Read the model definition and answer for the solid it produces. Units are mm, in the model's axes. A direction names the side the tool comes from. Give positions to 0.01 mm unless a question says otherwise; leave off trailing zeros. Loops run counter-clockwise (first coordinate to the right, second up) from the corner with the lowest first, then second, coordinate; pieces in that order, holes last. Notation, with made-up numbers: (70, 65) - (126, 65) arc R31 cw to (126, 93) - close; hole circle Ø9 at (87.25, 89). An arc over 180 degrees is marked (long way). Write each question's results on one line, items separated by ' | '. Start each with the question number.
Q1. The part is cut by section A-A, the plane y = 5. Write down the section's boundary in (x, z) (3 decimals), plus the area to 3 significant figures.
Q2. Given pin 1 (1 mm diameter, centred on x = -8.5, y = -4.5, fed in from +Z), flat-ended and moving along its own axis, determine where the tip first touches the part or whether it passes through.
Q3. Find the intervals of material crossed by line 1 (Y direction, x = -5.5, z = 471.5) (3 decimals), in increasing order. Write a range as from..to.
Q4. Determine the mould class of faces 3 (the flat face through (0, -9.525, 375)), 4 (the flat face through (11, 0, 774.7)), 5 (the flat face through (-12.7, 0, 375)), 6 (the flat face through (-9.525, 0, 375)) for opening direction X: +X half, -X half, draft (parallel to the pull), parting line (faces both ways), or undercut.
Q5. The part is cut by section C-C, the plane z = 679. Write down the section's boundary in (x, y) (3 decimals), plus the area to 3 significant figures.
Q6. For faces 1 (the flat face through (0, 12.7, 375)), 2 (the flat face through (0, 9.525, 375)), determine the directions among +Z, -Z, +X, -X, +Y, -Y from which every point of the face is accessible in a straight line to the end or side of a thin tool.
Autodesk Inventor part; units mm, degrees
ref_plane "Start Plane" through (0, 0, -12.7) normal (0, 0, 1) x (1, 0, 0)
ref_plane "End Plane" through (0, 0, 774.7) normal (0, 0, 1) x (1, 0, 0)
ref_plane "Work Plane5" through (0, 12.7, -12.7) normal (0, 0, -1) x (-1, 0, 0)
ref_plane "Start Plane" through (0, 0, -12.7) normal (0, 0, 1) x (1, 0, 0)
ref_plane "End Plane" through (0, 0, 774.7) normal (0, 0, 1) x (1, 0, 0)
sketch "Sketch" plane through (0, 0, 0) normal (0, 0, 1) x (1, 0, 0)
  line L0 (-12.7, 12.7) -> (12.7, 12.7)
  line L1 (12.7, 12.7) -> (12.7, -12.7)
  line L2 (12.7, -12.7) -> (-12.7, -12.7)
  line L3 (-12.7, -12.7) -> (-12.7, 12.7)
  line L4 (9.525, 9.525) -> (-9.525, 9.525)
  line L5 (-9.525, 9.525) -> (-9.525, -9.525)
  line L6 (-9.525, -9.525) -> (9.525, -9.525)
  line L7 (9.525, -9.525) -> (9.525, 9.525)
  point P0 (0, 0)
  point P1 (0, 12.7)
  point P2 (-12.7, 0)
  dimension "width" = 25.4
  dimension "d1" = 3.175
extrude "Body" add sketch "Sketch" along normal up to surface (787.4 mm away) from surface at -12.7
sketch "Sketch4" plane through (0, 0, 0) normal (0, 0, 1) x (1, 0, 0)
  line L0 (0, 0) -> (10, 0)
ref_plane "Work Plane4" through (0, 0, 0) normal (0, -1, 0) x (1, 0, 0)
sketch "Sketch5" plane through (0, 0, 0) normal (0, -1, 0) x (1, 0, 0)
  line L0 (-2, -12.7) -> (12, -12.7)
  line L1 (-2, 774.7) -> (12, 774.7)
  dimension "d9" = 787.4
ref_plane "Work Plane5" through (0, 12.7, -12.7) normal (0, 0, -1) x (-1, 0, 0)
split "Split1" plane through (0, 12.7, -12.7) removes the side toward (0, 0, -1)
ref_plane "Work Plane6" through (254, 12.7, 774.7) normal (0, 0, 1) x (1, 0, 0)
split "Split2" plane through (254, 12.7, 774.7) removes the side toward (0, 0, 1)
equation "\"G_OFFSET_START\" = 12.7"
equation "\"G_OFFSET_END\" = 12.7"
equation "\"d4\" = -G_OFFSET_START"
equation "\"d5\" = length + G_OFFSET_END"
equation "\"G_L\" = 762"
properties part number "Square Tube Profile" material "Aluminum-6061"
Check sheet entries:
1) outline: (-12.7, -12.7) - (-9.525, -12.7) - (-9.525, 774.7) - (-12.7, 774.7) - close; (9.525, -12.7) - (12.7, -12.7) - (12.7, 774.7) - (9.525, 774.7) - close | area: 5,000 mm^2
2) pin 1: passes through
3) line 1: y = -12.7..-9.525, 9.525..12.7
4) face 3: undercut | face 4: draft | face 5: -X half | face 6: undercut
5) outline: (-12.7, -12.7) - (12.7, -12.7) - (12.7, 12.7) - (-12.7, 12.7) - close; hole (-9.525, -9.525) - (9.525, -9.525) - (9.525, 9.525) - (-9.525, 9.525) - close | area: 282 mm^2
6) face 1: +Z, -Z, +X, -X, +Y | face 2: +Z, -Z
